Model file for the job. Use its own axes, mm. Give positions to 0.01 mm unless a question says otherwise; leave off trailing zeros. Write each loop counter-clockwise with the first axis right and the second up, starting at its lowest first coordinate (ties: lowest second). Pieces come first, ordered by that corner, then holes.
```python
from build123d import *

# Parameters (mm, degrees)
SKETCH_R           = 35.625
PAD_DEPTH          = 5
SKETCH001_R        = 2.15
POCKET_DEPTH       = 5
POLARPATTERN_COUNT = 4
CHAMFER_SIZE       = 1


with BuildPart() as part:
    # Sketch → Pad (new body)
    with BuildSketch(Plane.XY):
        Circle(SKETCH_R)
    extrude(amount=PAD_DEPTH)

    # Sketch001 → Pocket (cut)
    with BuildSketch(Plane.XY):
        with Locations((-21.995853, 20.40055)):
            Circle(SKETCH001_R)
    pocket = extrude(amount=POCKET_DEPTH, mode=Mode.SUBTRACT)

    # PolarPattern: Pocket ×4 about axis
    polarpattern_axis = Axis((0, 0, 0), (0, 0, 1))
    for i in range(1, POLARPATTERN_COUNT):
        add(pocket.rotate(polarpattern_axis, i * 360 / POLARPATTERN_COUNT), mode=Mode.SUBTRACT)

    # Chamfer
    chamfer_edges = [part.edges().sort_by_distance(p)[0] for p in [
        (24.145853, -20.40055, 5),
        (20.40055, 24.145853, 5),
        (-24.145853, 20.40055, 5),
        (-20.40055, -24.145853, 5),
    ]]
    chamfer(chamfer_edges, length=CHAMFER_SIZE)


solid = part.part
```
1. Slice it at C-C, the plane y = 8. Write the cut outline in (x, z), and give its area (3 significant figures).
Calculated:
outline: (-34.72, 0) - (34.72, 0) - (34.72, 5) - (-34.72, 5) - close
area: 347 mm2
2. Probe probe 1 along X at (y, z) = (21, 1.45); probe 2 along X at (y, z) = (-22, 1.9); probe 3 along X at (y, z) = (-18.5, 1). List the from-to ranges inside material, lowest first.
Calculated:
probe 1: x = -28.78 to -24.06, -19.93 to 18.5, 22.31 to 28.78
probe 2: x = -28.02 to -22.55, -18.25 to 20.56, 23.43 to 28.02
probe 3: x = -30.44 to 20.99, 23 to 30.44
3. Pull direction X, two halves, no side cores. Call faces 1 (the flat face through (0, 0, 0)), 2 (the cylindrical face through (-26.257, 24.077, 2.465)), 3 (the cylindrical face through (22.46, -18.3, 1.97)): +X half, -X half, draft (parallel to the pull), parting line (faces both ways), or undercut.
Calculated:
face 1: draft
face 2: parting line
face 3: undercut
4. Pin check, flat tips, straight feed: P1, Ø1, axis at x = 27.5, z = 4, coming from the -Y side; P2, Ø3, axis at x = 0.5, z = 2.5, coming from the +Y side (3 decimals); P3, Ø3, axis at y = 8.5, z = 2, coming from the -X side. Stop position of each tip, or through.
Calculated:
P1: stops at y = -23.24
P2: stops at y = 35.625
P3: stops at x = -34.93
5. Slice it at A-A, the plane z = 3.2. Write the cut outline in (x, y) (3 decimals).
Calculated:
outline: circle Ø71.25 at (0, 0); hole circle Ø4.3 at (-21.996, 20.401); hole circle Ø4.3 at (-20.401, -21.996); hole circle Ø4.3 at (20.401, 21.996); hole circle Ø4.3 at (21.996, -20.401)
6. Slice it at B-B, the plane x = -15. Write the cut outline in (y, z).
Calculated:
outline: (-32.31, 0) - (32.31, 0) - (32.31, 5) - (-32.31, 5) - close
